Drawing for the job (mm, zero at the part's lowest x, y, z). A direction names the side the tool comes from. Round coordinates to 2 decimals unless told otherwise and drop trailing zeros. Write each loop counter-clockwise with the first axis right and the second up, starting at its lowest first coordinate (ties: lowest second). Pieces come first, ordered by that corner, then holes.
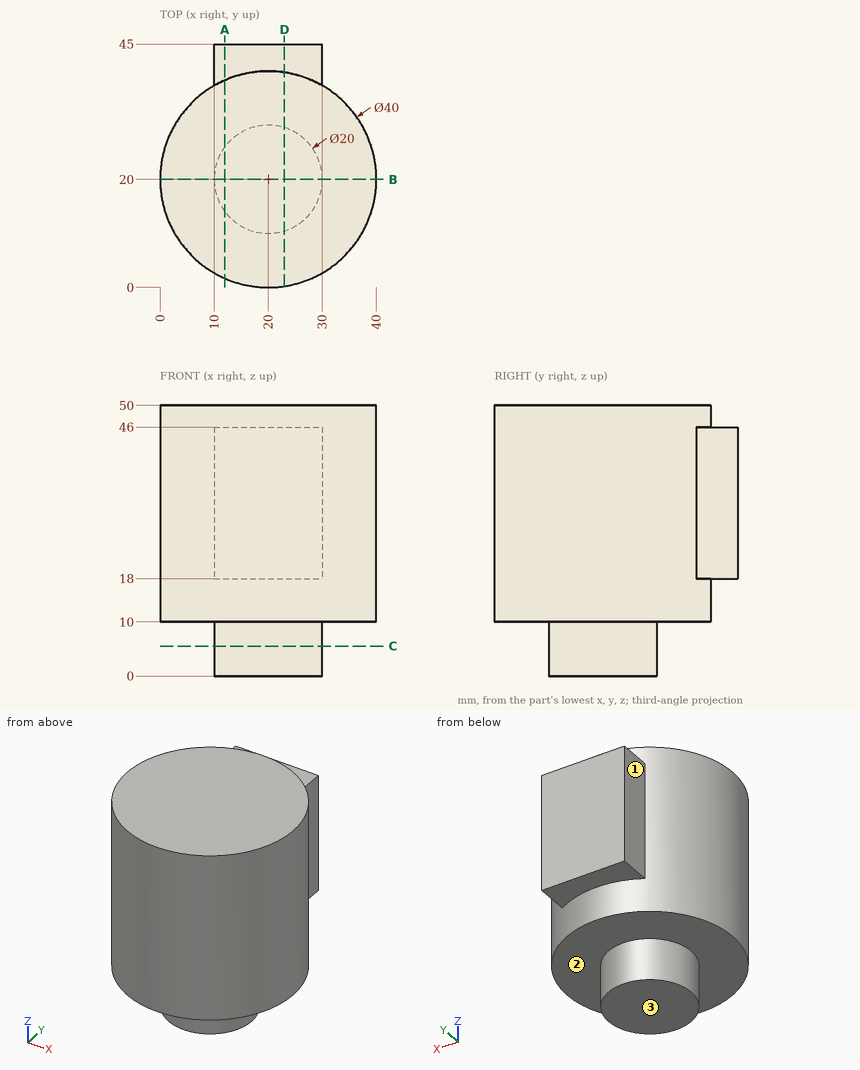
1) Flat gauge pins, fed straight in: pin 1 Ø6 at (y, z) = (40.5, 31.5) entering from +X; pin 2 Ø1.5 at (x, z) = (32, 33.5) entering from -Y; pin 3 Ø6 at (x, y) = (34, 37.5) entering from -Z. Where does each tip first touch, or does it go through?
2) Cut at D-D on x = 23. List the corners of the cut face in (y, z).
3) Which spindle directions (+Z, -Z, +X, -X, +Y, -Y) get a long thin tool onto all of the face, cutting with end or side? Do the marked faces 1, 2 and 3. Say none if no direction does.
4) Cut at C-C on z = 5.5. List the corners of the cut face in (x, y), and give its area (3 significant figures).
5) Cut at A-A on x = 12. List the corners of the cut face in (y, z).
6) Cut at B-B on y = 20. List the corners of the cut face in (x, z).
7) Wall check: probe 1 along Z at (x, y) = (28, 10); probe 2 along X at (y, z) = (41, 26); probe 3 along Z at (x, y) = (15, 43). Give the ranges that are in metal, low to high.
Result sheet:
1. pin 1: stops at x = 30
1. pin 2: stops at y = 3.46
1. pin 3: stops at z = 10
2. outline: (0.23, 10) - (10.46, 10) - (10.46, 0) - (29.54, 0) - (29.54, 10) - (39.77, 10) - (39.77, 18) - (45, 18) - (45, 46) - (39.77, 46) - (39.77, 50) - (0.23, 50) - close
3. face 1: +Z, -Z, -X, +Y
3. face 2: -Z
3. face 3: -Z, +X, -X, +Y, -Y
4. outline: circle Ø20 at (20, 20)
4. area: 314 mm2
5. outline: (1.67, 10) - (14, 10) - (14, 0) - (26, 0) - (26, 10) - (38.33, 10) - (38.33, 18) - (45, 18) - (45, 46) - (38.33, 46) - (38.33, 50) - (1.67, 50) - close
6. outline: (0, 10) - (10, 10) - (10, 0) - (30, 0) - (30, 10) - (40, 10) - (40, 50) - (0, 50) - close
7. probe 1: z = 10 to 50
7. probe 2: x = 10 to 30
7. probe 3: z = 18 to 46
